Check sheet for the drawn part. Datum: minimum x, y, z corner. Units: mm. A direction names the side the tool comes from. Round coordinates to 2 decimals unless told otherwise and drop trailing zeros. Loops run counter-clockwise (first coordinate to the right, second up) from the corner with the lowest first, then second, coordinate; pieces in that order, holes last.
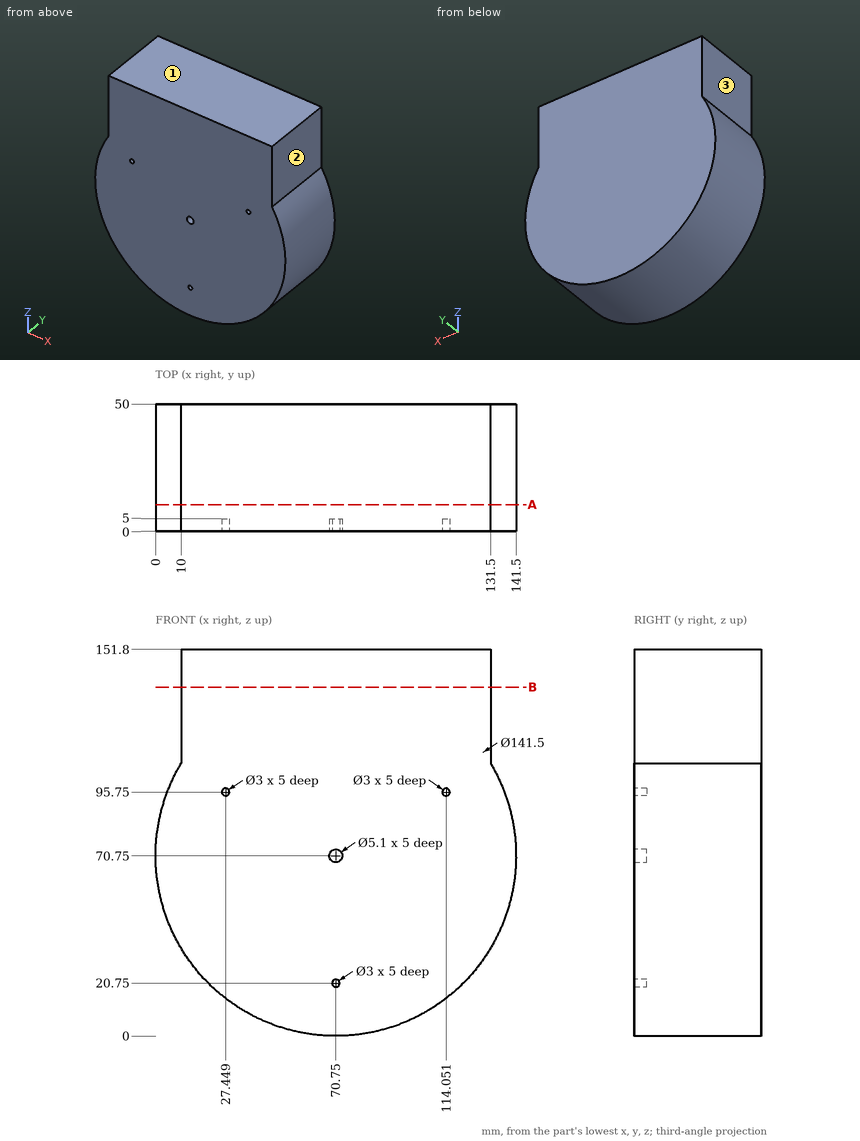
1) Access from +Z, -Z, +X, -X, +Y, -Y to the whole of each face (thin tool, end or side, straight path). Record for the marked faces 1, 2 and 3.
Report:
face 1: +Z, +X, -X, +Y, -Y
face 2: +Z, +X, +Y, -Y
face 3: +Z, -X, +Y, -Y
2) Sectioned sample at B-B, the plane z = 137. Record the cut outline in (x, y).
Report:
outline: (10, 0) - (131.5, 0) - (131.5, 50) - (10, 50) - close
3) Gauge pin test, flat ends, axial feed: pin 1 (4 mm diameter, centred on y = 37, z = 50.5, fed in from -X); pin 2 (8 mm diameter, centred on x = 85.5, y = 43, fed in from -Z); pin 3 (2 mm diameter, centred on x = 112.5, y = 37, fed in from -Z). Record the tip position at first contact, or that the pin passes through.
Report:
pin 1: stops at x = 2.39
pin 2: stops at z = 0.82
pin 3: stops at z = 12.91
4) Sectioned sample at A-A, the plane y = 10.5. Record the cut outline in (x, z).
Report:
outline: (10, 107.01) arc R70.75 ccw (long way) to (131.5, 107.01) - (131.5, 151.8) - (10, 151.8) - close
5) Scan lines: line 1 along X through (y, z) = (2.3, 95.75) (1 decimal); line 2 along X through (y, z) = (24, 143); line 3 along Z through (x, y) = (125.5, 27). Record each from-to range of solid material in increasing order.
Report:
line 1: x = 4.6 to 25.9, 28.9 to 112.6, 115.6 to 136.9
line 2: x = 10 to 131.5
line 3: z = 25.94 to 151.8
